from build123d import *

# Parameters (mm, degrees)
SKETCH1_R               = 6.35
BOSS_EXTRUDE1_DEPTH     = 69.85
SKETCH2_W               = 57.15
SKETCH2_H               = 54.522023849
CUT_EXTRUDE1_DEPTH      = 1
CUT_EXTRUDE1_DEPTH_BACK = 64.5


with BuildPart() as part:
    # Sketch1 → Boss-Extrude1 (new body)
    with BuildSketch(Plane.XY):
        with BuildLine():
            Line((-22.713461538, -22.102884615), (-22.713461538, -47.502884615))
            Line((-22.713461538, -47.502884615), (40.786538462, -47.502884615))
            Line((40.786538462, -47.502884615), (40.786538462, -22.102884615))
            ThreePointArc((40.786538462, -22.102884615), (9.036538462, 9.647115385), (-22.713461538, -22.102884615))
        make_face()
        with Locations((9.036538462, -6.227884615)):
            Circle(SKETCH1_R, mode=Mode.SUBTRACT)
    extrude(amount=BOSS_EXTRUDE1_DEPTH)

    # Sketch2 → Cut-Extrude1 (cut, two sides)
    with BuildSketch(Plane.ZY.offset(22.713461538)) as cut_extrude1_sk:
        with Locations((34.925, -13.891872691)):
            Rectangle(SKETCH2_W, SKETCH2_H)
    extrude(amount=CUT_EXTRUDE1_DEPTH, mode=Mode.SUBTRACT)
    extrude(cut_extrude1_sk.sketch, amount=-CUT_EXTRUDE1_DEPTH_BACK, mode=Mode.SUBTRACT)


solid = part.part
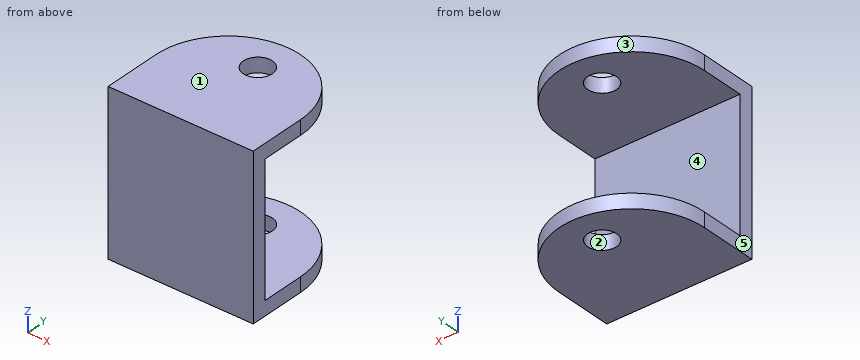
Design review of the part built by this model. Coordinates are the model's own, in mm. Face numbers are marked on the shaded views. A direction names the side the tool comes from. Give positions to 0.01 mm unless a question says otherwise; leave off trailing zeros. Write each loop counter-clockwise with the first axis right and the second up, starting at its lowest first coordinate (ties: lowest second). Pieces come first, ordered by that corner, then holes. Notation, with made-up numbers: M 79.5,69 L 92.5,69 A12 cw 92.5,91 Z; hole C 14.5,25.25 d3. An arc over 180 degrees is marked long. Return JSON: item names as keys, results as strings. Group by question number.
Item 1: Wall thickness on line 1 along Z through (x, y) = (2.5, -5); line 2 along Y through (x, z) = (-20, 12.5); line 3 along Y through (x, z) = (-3.5, 4.5): over which ranges is each line inside the solid? List them lowest first.
Item 2: Take a section at A-A (y = -31). Give the boundary of the cut face in (x, z).
Item 3: Tool access review of the marked faces 4 and 5: name each direction out of +Z, -Z, +X, -X, +Y, -Y from which nothing blocks a thin tool from reaching the whole face with its end or side.
Item 4: Take a section at D-D (z = 19.5). Give the boundary of the cut face in (x, y), plus the area to 3 significant figures.
Item 5: The part is to be moulded in two halves that separate along X. For the marked faces 1, 2 and 3, say which applies: pulls with the +X half, pulls with the -X half, needs draft (parallel to the pull), parting line crosses it, or undercut.
Item 6: Take a section at C-C (y = -3.5). Give the boundary of the cut face in (x, z).
Item 7: Clearance check with a flat-ended pin moving along its axis: pin 1 Ø10 at (x, y) = (9.04, -6.23) entering from +Z. State where the tip first meets the part, or that it passes through.
Item 8: Take a section at B-B (x = 12). Give the boundary of the cut face in (y, z), plus the area to 3 significant figures.
Return value:
{
 "1": {"line 1": "z = 0 to 6.35, 63.5 to 69.85", "line 2": "y = -47.5 to -41.15", "line 3": "y = -47.5 to 7.07"},
 "2": {"outline": "M -22.71,0 L 40.79,0 L 40.79,6.35 L -22.71,6.35 Z; M -22.71,63.5 L 40.79,63.5 L 40.79,69.85 L -22.71,69.85 Z"},
 "3": {"face 4": "+X, -X, +Y", "face 5": "+Z, -Z, -X, +Y, -Y"},
 "4": {"outline": "M -22.71,-47.5 L 40.79,-47.5 L 40.79,-41.15 L -22.71,-41.15 Z", "area": "403 mm2"},
 "5": {"face 1": "needs draft", "face 2": "undercut", "face 3": "parting line crosses it"},
 "6": {"outline": "M -16.69,0 L 3.3,0 L 3.3,6.35 L -16.69,6.35 Z; M -16.69,63.5 L 3.3,63.5 L 3.3,69.85 L -16.69,69.85 Z; M 14.77,0 L 34.77,0 L 34.77,6.35 L 14.77,6.35 Z; M 14.77,63.5 L 34.77,63.5 L 34.77,69.85 L 14.77,69.85 Z"},
 "7": {"pin 1": "passes through"},
 "8": {"outline": "M -47.5,0 L -11.84,0 L -11.84,6.35 L -41.15,6.35 L -41.15,63.5 L -11.84,63.5 L -11.84,69.85 L -47.5,69.85 Z; M -0.61,0 L 9.51,0 L 9.51,6.35 L -0.61,6.35 Z; M -0.61,63.5 L 9.51,63.5 L 9.51,69.85 L -0.61,69.85 Z", "area": "944 mm2"}
}
